Autodesk Inventor part; units mm, degrees
ref_plane "工作平面1" through (10, 18, 0) normal (-0.3643, -0.6585, -0.6585) x (0.875, 0, -0.4841)
ref_plane "YZ Plane" through (0, 0, 0) normal (1, 0, 0) x (0, 1, 0)
ref_plane "XZ Plane" through (0, 0, 0) normal (0, 1, 0) x (-1, 0, 0)
sketch "草圖1" plane through (0, 0, 0) normal (0, 1, 0) x (-1, 0, 0)
  line L0 (0, 0) -> (-57, 0)
  line L1 (-57, 0) -> (-57, -36)
  line L2 (-57, -36) -> (0, -36)
  line L3 (0, -36) -> (0, 0)
  dimension "d0" = 57
  dimension "d1" = 36
extrude "擠出1" add sketch "草圖1" along normal mid plane 36
sketch "草圖2" plane through (0, 18, 0) normal (0, 1, 0) x (1, 0, 0)
  line L0 (0, 0) -> (57, 0)
  line L1 (10, 0) -> (57, 6)
  line L2 (57, 0) -> (57, 36)
  dimension "d4" = 10
  dimension "d5" = 30
extrude "擠出2" cut sketch "草圖2" against normal blind 40
sketch "草圖3" plane through (57, -18, -36) normal (1, 0, 0) x (0, 0, -1)
  line L0 (-30, 16) -> (-10, 36)
  line L1 (0, 36) -> (-36, 36)
  line L2 (-30, 36) -> (-30, 0)
  point P0 (-36, 18)
  dimension "d8" = 20
  dimension "d9" = 20
ref_plane "工作平面1" through (10, 18, 0) normal (-0.3643, -0.6585, -0.6585) x (0.875, 0, -0.4841)
sketch "草圖4" plane through (10, 18, 0) normal (-0.3643, -0.6585, -0.6585) x (0.875, 0, -0.4841)
  line L0 (-15.1543, -12.3218) -> (93.717, -12.3218)
  line L1 (93.717, -12.3218) -> (93.717, 28.8166)
  line L2 (93.717, 28.8166) -> (-15.1543, 28.8166)
  line L3 (-15.1543, 28.8166) -> (-15.1543, -12.3218)
  point P0 (-8.7503, 10.3585)
extrude "擠出3" cut sketch "草圖4" against normal blind 40
mirror "鏡射1" about plane through (0, 0, 0) normal (0, 1, 0) of "擠出3"
properties part number "2"
The model under review builds one solid part; all positions refer to its coordinate system, in mm. Give positions to 0.01 mm unless a question says otherwise; leave off trailing zeros. Loops run counter-clockwise (first coordinate to the right, second up) from the corner with the lowest first, then second, coordinate; pieces in that order, holes last. Notation, with made-up numbers: (-21.5, 33.5) -> (-3.5, 33.5) arc R30 cw to (-3.5, 56.5) -> close; hole circle Ø2 at (40.5, -25.75). An arc over 180 degrees is marked (long way). Write each question's results on one line, items separated by ' | '.
1) Take a section at A-A, the plane y = 9. Give the boundary of the cut face in (x, z).
Conclusion:
outline: (0, -36) -> (57, -36) -> (57, -17) -> (31.14, -2.7) -> (10, 0) -> (0, 0) -> close
2) Insertion check: pin 1 Ø4 at (y, z) = (5.5, -14.5) entering from -X. The pin has a flat end and moves straight along its axis. Give the tip position at first contact, or say it passes through.
Conclusion:
pin 1: stops at x = 0
3) For line 1 along Y through (x, z) = (37, -9); line 2 along Z through (x, y) = (28.5, -10); line 3 along Z through (x, y) = (49.5, 12.5), list the stretches that pass through material, from the lowest coordinate up. Write a range as from..to.
Conclusion:
line 1: y = -12.06..12.06 | line 2: z = -36..-2.36 | line 3: z = -36..-16.36
4) Take a section at B-B, the plane x = 48. Give the boundary of the cut face in (y, z), plus the area to 3 significant figures.
Conclusion:
outline: (-18, -36) -> (18, -36) -> (18, -21.03) -> (1.83, -4.85) -> (-1.83, -4.85) -> (-18, -21.03) -> close | area: 860 mm^2
